Geometry: see drawing. Coordinates: mm, zero at the bounding-box minimum. A direction names the side the tool comes from. Round coordinates to 2 decimals unless told otherwise and drop trailing zeros. Loops run counter-clockwise (first coordinate to the right, second up) from the corner with the lowest first, then second, coordinate; pieces in that order, holes last.
(1) Access query for the marked faces 1 and 2. Directions: +Z, -Z, +X, -X, +Y, -Y. A direction counts if a zero-diameter tool reaches every point of the face in a straight line with its end or side. Return the directions, or none.
(2) Line query: line 1 (Y direction, x = 12.75, z = 125); line 2 (X direction, y = 13, z = 100.5); line 3 (Y direction, x = 166.5, z = 76.5) (1 decimal). Output: solid intervals per line, ascending.
(3) Cut plane D-D, the plane y = 44. Output: boundary loops of the cut face in (x, z) (1 decimal), and give its area (3 significant figures).
(4) Cut plane C-C, the plane x = 171.5. Output: boundary loops of the cut face in (y, z), and give its area (3 significant figures).
(5) Cut plane A-A, the plane z = 25. Output: boundary loops of the cut face in (x, y), and give its area (3 significant figures).
(6) First-contact query: pin 1 Ø1.5 at (y, z) = (202.5, 37) entering from +X; pin 2 Ø6 at (x, y) = (72, 157.5) entering from -Z; pin 3 Ø4 at (x, z) = (92, 129.5) entering from +Y (1 decimal). Flat tips, straight axial feed; report the tip coordinate or a pass-through.
(7) Cut plane B-B, the plane z = 125. Output: boundary loops of the cut face in (x, y), and give its area (3 significant figures).
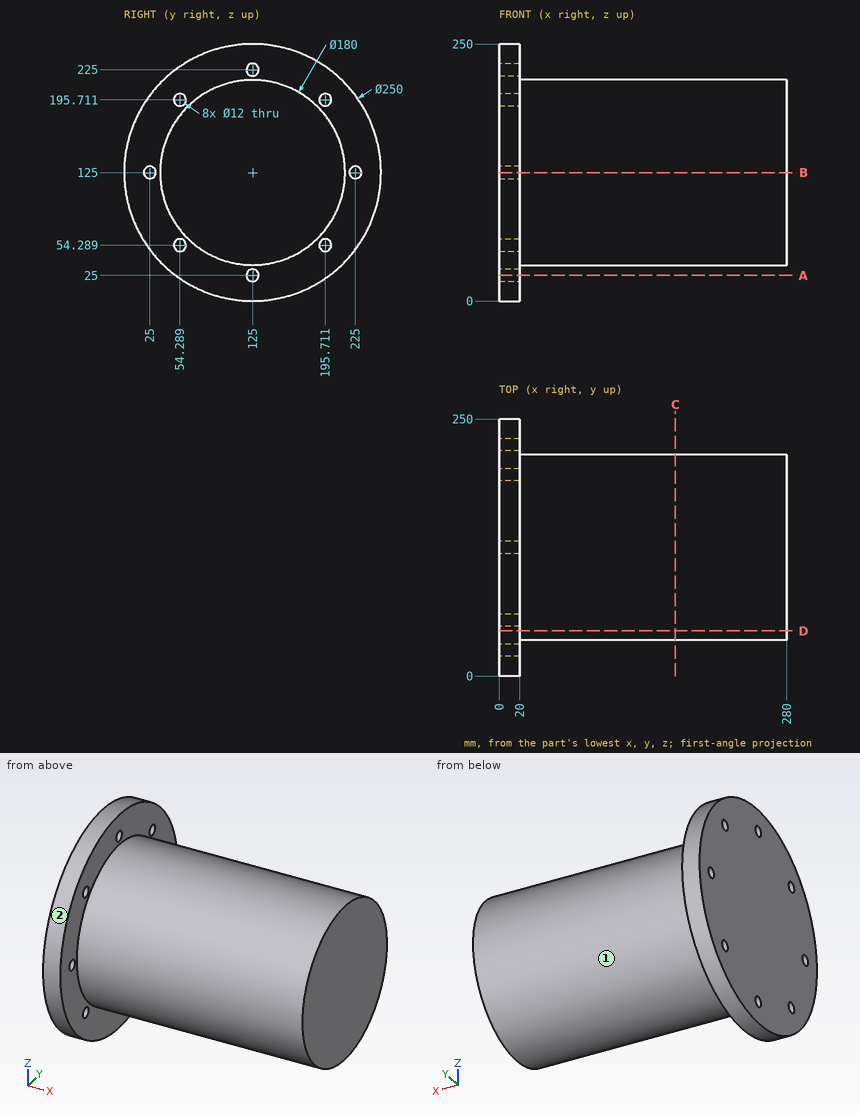
Reported:
1. face 1: +X
1. face 2: +X, -X
2. line 1: y = 0 to 19, 31 to 219, 231 to 250
2. line 2: x = 0 to 20
2. line 3: y = 49.2 to 200.8
3. outline: (0, 29.8) - (20, 29.8) - (20, 85.8) - (280, 85.8) - (280, 164.2) - (20, 164.2) - (20, 220.2) - (0, 220.2) - close
3. area: 24,200 mm2
4. outline: circle Ø180 at (125, 125)
4. area: 25,400 mm2
5. outline: (0, 50) - (20, 50) - (20, 119) - (0, 119) - close; (0, 131) - (20, 131) - (20, 200) - (0, 200) - close
5. area: 2,760 mm2
6. pin 1: stops at x = 20
6. pin 2: stops at z = 39.97
6. pin 3: stops at y = 215
7. outline: (0, 0) - (20, 0) - (20, 19) - (0, 19) - close; (0, 31) - (20, 31) - (20, 35) - (280, 35) - (280, 215) - (20, 215) - (20, 219) - (0, 219) - close; (0, 231) - (20, 231) - (20, 250) - (0, 250) - close
7. area: 51,300 mm2
